Source: CAD feature listing. Evaluate the final solid. Frame: model axes, mm. A direction names the side the tool comes from. Give positions to 0.01 mm unless a question says otherwise; leave off trailing zeros. Order: outer loops, then holes, each group sorted by start corner. A loop starts at its lowest first (then second) coordinate and runs counter-clockwise, first axis right, second up. Notation, with made-up numbers: M -25.75,-11.5 L -7.75,-11.5 A20 ccw -7.75,1.5 Z; hole C 49,82 d8. An arc over 180 degrees is marked long. Return JSON: item names as keys, results as strings.
from build123d import *

# Parameters (mm, degrees)
CROQUIS8_W            = 2.174939389
CROQUIS8_H            = 2.19283881
CORTAR_EXTRUIR2_DEPTH = 10
CROQUIS11_R           = 1
CORTAR_EXTRUIR3_DEPTH = 9.185352772
CORTAR_EXTRUIR3_TAPER = 6
CROQUIS13_OUTSIDE_W   = 10.94
CROQUIS13_OUTSIDE_H   = 10.94
CORTAR_EXTRUIR4_DEPTH = 10


with BuildPart() as part:
    # Croquis1 → Revolución1 (revolve)
    with BuildSketch(Plane(origin=(0, 0, 0), x_dir=(1, 0, 0), z_dir=(0, 1, 0))):
        Polygon((2.5, 5), (0, 5), (0, 0), (2.5, 0), (2.5, 1), (3, 1), (3, 4.5), align=None)
    revolve(axis=Axis((0, 0, -5), (0, 0, 1)))

    # Croquis2 → Cortar-Revolución1 (revolve, cut)
    with BuildSketch(Plane(origin=(0, 0, 0), x_dir=(1, 0, 0), z_dir=(0, 1, 0))):
        Polygon((1.5, 5), (0, 5), (0, -8), (0.2, -8), (0.2, -7.2), (1, -6.4), (1, 4.5), align=None)
    revolve(axis=Axis((0, 0, -5), (0, 0, 1)), mode=Mode.SUBTRACT)

    # Croquis4 → Revolución2 (revolve)
    with BuildSketch(Plane(origin=(0, 0, 0), x_dir=(1, 0, 0), z_dir=(0, 1, 0)), mode=Mode.PRIVATE) as revoluci_n2_sk:
        Polygon((0, 0), (0, -8), (3, -4), (3, 0), align=None)
    revolve(revoluci_n2_sk.sketch.rotate(Axis((0, 0, 0), (0, 0, 1)), 180), axis=Axis((0, 0, 0), (0, 0, 1)))

    # Croquis8 → Cortar-Extruir2 (cut)
    with BuildSketch(Plane.XY.offset(7)):
        with Locations((-0.052168773, -0.007828758)):
            Rectangle(CROQUIS8_W, CROQUIS8_H)
    extrude(amount=CORTAR_EXTRUIR2_DEPTH, mode=Mode.SUBTRACT)

    # Croquis11 → Cortar-Extruir3 (cut, through all)
    with BuildSketch(Plane.XY):
        Circle(CROQUIS11_R)
    extrude(amount=CORTAR_EXTRUIR3_DEPTH, taper=CORTAR_EXTRUIR3_TAPER, mode=Mode.SUBTRACT)

    # Croquis13 outside → Cortar-Extruir4 (cut)
    with BuildSketch(Plane.XY):
        Rectangle(CROQUIS13_OUTSIDE_W, CROQUIS13_OUTSIDE_H)
        Polygon((2.763390844, 1.167763265), (0.370382769, 2.977048304), (-2.393008075, 1.809285039), (-2.763390844, -1.167763265), (-0.370382769, -2.977048304), (2.393008075, -1.809285039), align=None, mode=Mode.SUBTRACT)
    extrude(amount=CORTAR_EXTRUIR4_DEPTH, mode=Mode.SUBTRACT)


solid = part.part
1. Section query C-C (z = 2). Return loops of the section in (x, y).
Evaluation:
{"outline": "M -2.76,-1.17 L -0.37,-2.98 L 2.39,-1.81 L 2.76,1.17 L 0.37,2.98 L -2.39,1.81 Z; hole C 0,0 d1.58"}
2. Section query A-A (y = 0). Return loops of the section in (x, z), then the cut area to 3 significant figures.
Evaluation:
{"outline": "M -3,-4.5 L -2.5,-5 L -1.5,-5 L -1,-4.5 L -1,0 L -0.26,7 L -0.75,7 L -2.62,4.51 L -2.62,0 L -2.5,0 L -2.5,-1 L -3,-1 Z; M 0.26,7 L 1,0 L 1,-4.5 L 1.5,-5 L 2.5,-5 L 3,-4.5 L 3,-1 L 2.5,-1 L 2.5,0 L 2.62,0 L 2.62,4.51 L 0.75,7 Z", "area": "41.7 mm^2"}
3. Ray query, probe 1 along Y at (x, z) = (0, -3.1); probe 2 along X at (y, z) = (0.1, 4.25); probe 3 along X at (y, z) = (0.35, 2.75). Return the intervals inside material, ascending.
Evaluation:
{"probe 1": "y = -3 to -1, 1 to 3", "probe 2": "x = -2.61 to -0.54, 0.54 to 2.63", "probe 3": "x = -2.57 to -0.62, 0.62 to 2.66"}
4. Draft query along Y for faces 1 (the face through (-0.08, 0.62, 3.55)), 2 (the face through (2, 2, -1)), 3 (the face through (0, -1, -2)), 4 (the face through (-1, 2.4, 2.2)). Return one class per face: pulls with the +Y half, pulls with the -Y half, needs draft (parallel to the pull), parting line crosses it, or undercut.
Evaluation:
{"face 1": "undercut", "face 2": "needs draft", "face 3": "undercut", "face 4": "pulls with the +Y half"}
5. Section query B-B (x = 0). Return loops of the section in (y, z), then the cut area to 3 significant figures.
Evaluation:
{"outline": "M -3,-4.5 L -2.5,-5 L -1.5,-5 L -1,-4.5 L -1,0 L -0.26,7 L -0.75,7 L -2.82,4.24 L -2.82,0 L -2.5,0 L -2.5,-1 L -3,-1 Z; M 0.26,7 L 1,0 L 1,-4.5 L 1.5,-5 L 2.5,-5 L 3,-4.5 L 3,-1 L 2.5,-1 L 2.5,0 L 2.82,0 L 2.82,4.24 L 0.75,7 Z", "area": "43.4 mm^2"}
6. Section query D-D (z = 3.25). Return loops of the section in (x, y), then the cut area to 3 significant figures.
Evaluation:
{"outline": "M -2.76,-1.17 L -0.37,-2.98 L 2.39,-1.81 L 2.76,1.17 L 0.37,2.98 L -2.39,1.81 Z; hole C 0,0 d1.32", "area": "22.0 mm^2"}
7. First-contact query: pin 1 (1.2 mm diameter, centred on x = 0, y = 0, fed in from +Z); pin 2 (1.5 mm diameter, centred on x = -1, z = -1, fed in from +Y). Flat tips, straight axial feed; report the tip coordinate or a pass-through.
Evaluation:
{"pin 1": "stops at z = 7", "pin 2": "stops at y = 2.99"}
8. Set-up query: faces 5 (the face through (-1.58, -2.06, 2.24)), 6 (the face through (1.58, 2.06, 2.24)), 7 (the face through (2.576, -0.342, 2.236)). Return all of +Z, -Z, +X, -X, +Y, -Y with unobstructed straight access to the full face (end or side cutting, diameter ignored); none if empty.
Evaluation:
{"face 5": "+Z, -X, -Y", "face 6": "+Z, +X, +Y", "face 7": "+Z, +X, -Y"}
